```python
from build123d import *

# Parameters (mm, degrees)
F1_DEPTH = 6
F2_DEPTH = 8


with BuildPart() as f1:
    # F0 (on Top) → F1 (new body)
    with BuildSketch(Plane.XY):
        Polygon((31.226261, 74.712449), (1.234041, 17.045589), (3.234041, 17.045589), (33.226261, 74.712449), align=None)
        with BuildLine():
            Line((3.234041, 17.045589), (1.234041, 17.045589))
            ThreePointArc((1.234041, 17.045589), (0.445743, 14.923822), (0.201795, 12.673533))
            Line((0.201795, 12.673533), (2, 13.549008))
            ThreePointArc((2, 13.549008), (2.494165, 15.340658), (3.234041, 17.045589))
        make_face()
    extrude(amount=F1_DEPTH)

    # F0 (on Top) → F2 (join)
    with BuildSketch(Plane.XY):
        Polygon((31.226261, 74.712449), (1.234041, 17.045589), (3.234041, 17.045589), (33.226261, 74.712449), align=None)
        with BuildLine():
            Line((3.234041, 17.045589), (1.234041, 17.045589))
            ThreePointArc((1.234041, 17.045589), (0.445743, 14.923822), (0.201795, 12.673533))
            Line((0.201795, 12.673533), (2, 13.549008))
            ThreePointArc((2, 13.549008), (2.494165, 15.340658), (3.234041, 17.045589))
        make_face()
    extrude(amount=F2_DEPTH)


solid = f1.part
```
Geometry: final body of the model. Coordinates: model frame, mm. Give positions to 0.01 mm unless a question says otherwise; leave off trailing zeros. Loops run counter-clockwise (first coordinate to the right, second up) from the corner with the lowest first, then second, coordinate; pieces in that order, holes last. Notation, with made-up numbers: (-35, 22.5) -> (-1, 22.5) arc R14 ccw to (-1, 36.5) -> close; hole circle Ø8 at (70.5, -37.5). An arc over 180 degrees is marked (long way). Use CSV: the item, a comma, the result in double quotes.
(1) Ray query, line 1 along Y through (x, z) = (27.5, 1); line 2 along X through (y, z) = (53, 4); line 3 along Y through (x, z) = (31.5, 7). Return the intervals inside material, ascending. Write a range as [from, to].
From the geometry:
line 1,"[63.7, 67.55]"
line 2,"[19.93, 21.93]"
line 3,"[71.39, 74.71]"
(2) Cut plane C-C (y = 51). Output: boundary loops of the cut face in (x, z), plus the area to 3 significant figures.
From the geometry:
outline,"(18.89, 0) -> (20.89, 0) -> (20.89, 8) -> (18.89, 8) -> close"
area,"16.0 mm^2"
(3) Cut plane A-A (z = 6.5). Output: boundary loops of the cut face in (x, y), plus the area to 3 significant figures.
From the geometry:
outline,"(0.2, 12.67) -> (2, 13.55) arc R13.26 cw to (3.23, 17.05) -> (33.23, 74.71) -> (31.23, 74.71) -> (1.23, 17.05) arc R9.16 ccw to start"
area,"123 mm^2"
(4) Cut plane B-B (x = 28.5). Output: boundary loops of the cut face in (y, z).
From the geometry:
outline,"(65.63, 0) -> (69.47, 0) -> (69.47, 8) -> (65.63, 8) -> close"
(5) First-contact query: P1, Ø3, axis at y = 58.5, z = 3, coming from the -X side; P2, Ø3, axis at y = 31, z = 6.5, coming from the -X side; P3, Ø1.5, axis at x = 6.5, z = 7, coming from the -Y side. Flat tips, straight axial feed; report the tip coordinate or a pass-through.
From the geometry:
P1,"x = 22.01"
P2,"x = 7.71"
P3,"y = 21.88"
